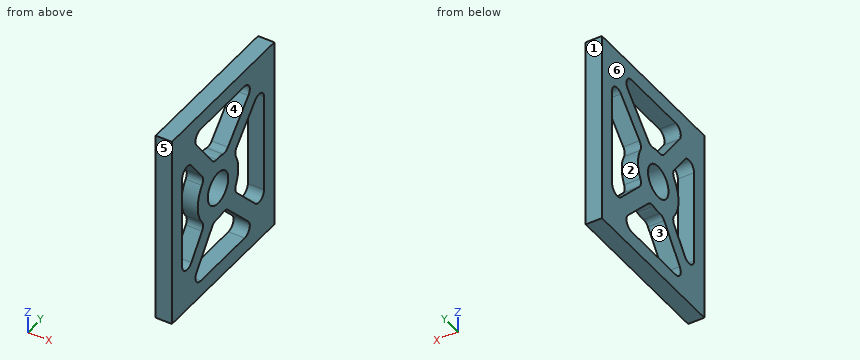
```python
from build123d import *

# Parameters (mm, degrees)
SKETCH1_W           = 76.2
SKETCH1_H           = 63.5
SKETCH1_R           = 6.35
BOSS_EXTRUDE1_DEPTH = 6.35
CUT_EXTRUDE1_REACH  = 54.074
FILLET2_R           = 3.175


with BuildPart() as part:
    # Sketch1 → Boss-Extrude1 (new body)
    with BuildSketch(Plane(origin=(0, 0, 0), x_dir=(0, 0, -1), z_dir=(1, 0, 0))):
        with Locations((0, 3.175)):
            Rectangle(SKETCH1_W, SKETCH1_H)
        Circle(SKETCH1_R, mode=Mode.SUBTRACT)
    extrude(amount=BOSS_EXTRUDE1_DEPTH)

    # Sketch4 → Cut-Extrude1 (cut, up to next)
    with BuildSketch(Plane(origin=(6.35, 0, 0), x_dir=(0, 0, -1), z_dir=(1, 0, 0)), mode=Mode.PRIVATE) as cut_extrude1_sk1:
        with BuildLine():
            Line((-9.415500655, -8.336066847), (-27.940897809, -22.225))
            Line((-27.940897809, -22.225), (27.940897809, -22.225))
            Line((27.940897809, -22.225), (9.415500655, -8.336066847))
            ThreePointArc((9.415500655, -8.336066847), (0, -12.575438882), (-9.415500655, -8.336066847))
        make_face()
    cut_extrude1_tool1 = extrude(cut_extrude1_sk1.sketch, amount=-CUT_EXTRUDE1_REACH, mode=Mode.PRIVATE) & part.part
    # Sketch4 → Cut-Extrude1 (cut, up to next)
    with BuildSketch(Plane(origin=(6.35, 0, 0), x_dir=(0, 0, -1), z_dir=(1, 0, 0)), mode=Mode.PRIVATE) as cut_extrude1_sk2:
        with BuildLine():
            Line((-12.310078524, -2.569752866), (-31.75, -17.144326768))
            Line((-31.75, -17.144326768), (-31.75, 23.984763034))
            Line((-31.75, 23.984763034), (-11.639261898, 4.761223113))
            ThreePointArc((-11.639261898, 4.761223113), (-12.523119774, 1.145920677), (-12.310078524, -2.569752866))
        make_face()
    cut_extrude1_tool2 = extrude(cut_extrude1_sk2.sketch, amount=-CUT_EXTRUDE1_REACH, mode=Mode.PRIVATE) & part.part
    # Sketch4 → Cut-Extrude1 (cut, up to next)
    with BuildSketch(Plane(origin=(6.35, 0, 0), x_dir=(0, 0, -1), z_dir=(1, 0, 0)), mode=Mode.PRIVATE) as cut_extrude1_sk3:
        with BuildLine():
            Line((-27.362264298, 28.575), (-7.793369677, 9.869399786))
            ThreePointArc((-7.793369677, 9.869399786), (0, 12.575438882), (7.793369677, 9.869399786))
            Line((7.793369677, 9.869399786), (27.362264298, 28.575))
            Line((27.362264298, 28.575), (-27.362264298, 28.575))
        make_face()
    cut_extrude1_tool3 = extrude(cut_extrude1_sk3.sketch, amount=-CUT_EXTRUDE1_REACH, mode=Mode.PRIVATE) & part.part
    # Sketch4 → Cut-Extrude1 (cut, up to next)
    with BuildSketch(Plane(origin=(6.35, 0, 0), x_dir=(0, 0, -1), z_dir=(1, 0, 0)), mode=Mode.PRIVATE) as cut_extrude1_sk4:
        with BuildLine():
            Line((31.75, 23.984763034), (11.639261898, 4.761223113))
            ThreePointArc((11.639261898, 4.761223113), (12.523119774, 1.145920677), (12.310078524, -2.569752866))
            Line((12.310078524, -2.569752866), (31.75, -17.144326768))
            Line((31.75, -17.144326768), (31.75, 23.984763034))
        make_face()
    cut_extrude1_tool4 = extrude(cut_extrude1_sk4.sketch, amount=-CUT_EXTRUDE1_REACH, mode=Mode.PRIVATE) & part.part
    add(cut_extrude1_tool1.solids().sort_by_distance((6.35, -17.188664, 0))[0], mode=Mode.SUBTRACT)
    add(cut_extrude1_tool2.solids().sort_by_distance((6.35, 2.651872, 24.218351))[0], mode=Mode.SUBTRACT)
    add(cut_extrude1_tool3.solids().sort_by_distance((6.35, 21.415116, 0))[0], mode=Mode.SUBTRACT)
    add(cut_extrude1_tool4.solids().sort_by_distance((6.35, 2.651872, -24.218351))[0], mode=Mode.SUBTRACT)

    # Fillet2
    fillet2_edges = [part.edges().sort_by_distance(p)[0] for p in [
        (3.175, 4.761223113, 11.639261898),
        (3.175, -2.569752866, 12.310078524),
        (3.175, -17.144326768, 31.75),
        (3.175, 23.984763034, 31.75),
        (3.175, -8.336066847, 9.415500655),
        (3.175, -8.336066847, -9.415500655),
        (3.175, -22.225, -27.940897809),
        (3.175, -22.225, 27.940897809),
        (3.175, 28.575, 27.362264298),
        (3.175, 28.575, -27.362264298),
        (3.175, 9.869399786, -7.793369677),
        (3.175, 9.869399786, 7.793369677),
        (3.175, 23.984763034, -31.75),
        (3.175, -17.144326768, -31.75),
        (3.175, -2.569752866, -12.310078524),
        (3.175, 4.761223113, -11.639261898),
    ]]
    fillet(fillet2_edges, radius=FILLET2_R)


solid = part.part
```
Source: CAD feature listing. Evaluate the final solid. Frame: model axes, mm. Face numbers are marked on the shaded views. A direction names the side the tool comes from. Coordinates: 2 decimals unless noted, no trailing zeros. Loops run counter-clockwise (first coordinate to the right, second up) from the corner with the lowest first, then second, coordinate; pieces in that order, holes last. Notation, with made-up numbers: M 18,50.25 L 23,50.25 A23 cw 23,87.25 Z; hole C 44,40 d4. An arc over 180 degrees is marked long. Use a Markdown table: item, result. Add a question column.
Q1. Draft query along Y for the marked faces 3, 4, 5 and 6. Return one class per face: pulls with the +Y half, pulls with the -Y half, needs draft (parallel to the pull), parting line crosses it, or undercut.
Q2. Section query C-C, the plane x = 4. State how many separate pieces and enclosed holes the cut face has, and give its area (3 significant figures).
Q3. Section query B-B, the plane z = 0. Return loops of the section in (x, y) (3 decimals), and give its area (3 significant figures).
Q4. First-contact query: pin 1 (1 mm diameter, centred on y = 12.5, z = 6.5, fed in from -X). Flat tip, straight axial feed; report the tip coordinate or a pass-through.
Q5. Material intervals for L1, parallel to Y at x = 4.25, z = 0 (3 decimals); L2, parallel to Y at x = 2.5, z = 18.5 (3 decimals); L3, parallel to Y at x = 5, z = -22 (3 decimals), sorted ascending.
Q6. Access query for the marked faces 1 and 2. Directions: +Z, -Z, +X, -X, +Y, -Y. A direction counts if a zero-diameter tool reaches every point of the face in a straight line with its end or side. Return the directions, or none.
Q7. Section query A-A, the plane y = 0. Return loops of the section in (x, z).
Result:
| question | item | result |
|---|---|---|
| 1 | face 3 | undercut |
| 1 | face 4 | undercut |
| 1 | face 5 | pulls with the -Y half |
| 1 | face 6 | needs draft |
| 2 | separate pieces | 1 |
| 2 | enclosed holes | 5 |
| 2 | area | 2,780 mm2 |
| 3 | outline | M 0,-28.575 L 6.35,-28.575 L 6.35,-22.225 L 0,-22.225 Z; M 0,-12.575 L 6.35,-12.575 L 6.35,-6.35 L 0,-6.35 Z; M 0,6.35 L 6.35,6.35 L 6.35,12.575 L 0,12.575 Z; M 0,28.575 L 6.35,28.575 L 6.35,34.925 L 0,34.925 Z |
| 3 | area | 160 mm2 |
| 4 | pin 1 | passes through |
| 5 | L1 | y = -28.575 to -22.225, -12.575 to -6.35, 6.35 to 12.575, 28.575 to 34.925 |
| 5 | L2 | y = -28.575 to -22.224, -15.147 to -7.21, 11.319 to 20.104, 28.575 to 34.925 |
| 5 | L3 | y = -28.575 to -9.835, 14.665 to 23.514, 27.286 to 34.925 |
| 6 | face 1 | +Z, -Z, +X, -X, +Y |
| 6 | face 2 | +X, -X |
| 7 | outline | M 0,-38.1 L 6.35,-38.1 L 6.35,-31.75 L 0,-31.75 Z; M 0,-12.58 L 6.35,-12.58 L 6.35,-6.35 L 0,-6.35 Z; M 0,6.35 L 6.35,6.35 L 6.35,12.58 L 0,12.58 Z; M 0,31.75 L 6.35,31.75 L 6.35,38.1 L 0,38.1 Z |
